```python
from build123d import *

# Parameters (mm, degrees)
F0_W          = 52
F0_H          = 1.2
F0_H_2        = 200.6
F1_DEPTH      = 50
F0_W_2        = 36.4451892475
F2_DEPTH      = 44
F0_W_3        = 531.5548107525
F3_DEPTH      = 30
F4_DEPTH      = 1.2
F5_R          = 1.2
F6_R          = 3
F7_W          = 30.6323694531
F7_H          = 5.0316524575
F8_DEPTH      = 25
F9_W          = 30.6323694531
F9_H          = 8.4860329516
F10_DEPTH     = 2
F11_T1_DEPTH  = 44.7745050768
F11_T6_DEPTH  = 22.6281685754
F11_T11_DEPTH = 22.6281685754


# Not quite as in the source:
# - a fillet or chamfer that OpenCascade refuses, or shapes differently, is made with other operations: its cross-section is extruded or revolved along the edge and cut away or added


with BuildPart() as f1:
    # F0 (on Top) → F1 (new body)
    with BuildSketch(Plane.XY):
        with Locations((-71.6174369702, 163.7731539965)):
            Rectangle(F0_W, F0_H)
        with Locations((-71.6174369702, 62.8731539965)):
            Rectangle(F0_W, F0_H_2)
        with Locations((-71.6174369702, -38.0268460035)):
            Rectangle(F0_W, F0_H)
    extrude(amount=F1_DEPTH)

    # F0 (on Top) → F2 (join)
    with BuildSketch(Plane.XY):
        with Locations((-27.3948423465, -38.0268460035)):
            Rectangle(F0_W_2, F0_H)
        with Locations((-27.3948423465, 163.7731539965)):
            Rectangle(F0_W_2, F0_H)
    extrude(amount=F2_DEPTH)

    # F0 (on Top) → F3 (join)
    with BuildSketch(Plane.XY):
        with Locations((256.6051576535, 163.7731539965)):
            Rectangle(F0_W_3, F0_H)
        with Locations((256.6051576535, -38.0268460035)):
            Rectangle(F0_W_3, F0_H)
    extrude(amount=F3_DEPTH)

    # F0 (on Top) → F4 (join)
    with BuildSketch(Plane.XY):
        with Locations((256.6051576535, 62.8731539965)):
            Rectangle(F0_W_3, F0_H_2)
        with Locations((-27.3948423465, 62.8731539965)):
            Rectangle(F0_W_2, F0_H_2)
    extrude(amount=F4_DEPTH)

    # F5
    f5_edges = [f1.edges().sort_by_distance(p)[0] for p in [
        (-71.617437, -38.626846, 50),
        (-71.617437, 164.373154, 50),
        (-97.617437, 62.873154, 50),
        (-97.617437, 62.873154, 0),
        (-45.617437, 62.873154, 50),
        (-45.617437, -38.026846, 44),
    ]]
    fillet(f5_edges, radius=F5_R)

    # F6
    f6_edges = [f1.edges().sort_by_distance(p)[0] for p in [
        (-9.172248, -38.026846, 44),
        (522.382563, -38.026846, 30),
        (522.382563, 163.773154, 30),
        (-9.172248, 163.773154, 44),
        (-9.172248, 163.773154, 30),
        (-9.172248, -38.026846, 30),
    ]]
    fillet(f6_edges, radius=F6_R)

    # F7 (on face) → F8 (cut)
    with BuildSketch(Plane.XZ.offset(-163.1731539965)):
        with Locations((11.9725436671, 3.6928627233)):
            Rectangle(F7_W, F7_H)
    extrude(amount=-F8_DEPTH, mode=Mode.SUBTRACT)

    # F9 (on face) → F10 (join)
    with BuildSketch(Plane.XZ.offset(-163.1731539965)):
        with Locations((11.9725436671, 10.4517054278)):
            Rectangle(F9_W, F9_H)
    extrude(amount=F10_DEPTH)

    # F11: fillet of radius 3 on 3 edges, made by hand

    # F11_s2 → F11_t1 (cut)
    with BuildSketch(Plane.YZ.offset(-10.4147088713)):
        with BuildLine():
            ThreePointArc((163.1731539965, 14.6947219037), (161.7236642537, 13.5983455865), (161.1731539965, 11.8662947789))
            Line((161.1731539965, 11.8662947789), (161.1731539965, 14.6947219037))
            Line((161.1731539965, 14.6947219037), (163.1731539965, 14.6947219037))
        make_face()
    extrude(amount=F11_T1_DEPTH, mode=Mode.SUBTRACT)


with BuildPart() as f11_tool4:
    # F11_s5 → F11_t6 (new body)
    with BuildSketch(Plane.XY.offset(-0.8623788598)):
        with BuildLine():
            ThreePointArc((27.2887283936, 163.1731539965), (26.1923520764, 161.7236642537), (24.4603012689, 161.1731539965))
            Line((24.4603012689, 161.1731539965), (27.2887283936, 161.1731539965))
            Line((27.2887283936, 161.1731539965), (27.2887283936, 163.1731539965))
        make_face()
    extrude(amount=F11_T6_DEPTH)

    split(bisect_by=Plane.XY.offset(1.2), keep=Keep.TOP)


with BuildPart() as f1_1:
    add(f1.part)

    # F11_t3: cut F11_tool4
    add(f11_tool4.part, mode=Mode.SUBTRACT)


with BuildPart() as f11_tool9:
    # F11_s10 → F11_t11 (new body)
    with BuildSketch(Plane.XY.offset(21.7657897155)):
        with BuildLine():
            ThreePointArc((-3.3436410595, 163.1731539965), (-2.2472647423, 161.7236642537), (-0.5152139347, 161.1731539965))
            Line((-0.5152139347, 161.1731539965), (-3.3436410595, 161.1731539965))
            Line((-3.3436410595, 161.1731539965), (-3.3436410595, 163.1731539965))
        make_face()
    extrude(amount=-F11_T11_DEPTH)

    split(bisect_by=Plane.XY.offset(1.2), keep=Keep.TOP)


with BuildPart() as f1_2:
    add(f1_1.part)

    # F11_t8: cut F11_tool9
    add(f11_tool9.part, mode=Mode.SUBTRACT)


solid = f1_2.part
```
Here's how the part is built. I have some questions about the finished solid (model axes, mm). A direction names the side the tool comes from. Give positions to 0.01 mm unless a question says otherwise; leave off trailing zeros. Write each loop counter-clockwise with the first axis right and the second up, starting at its lowest first coordinate (ties: lowest second). Pieces come first, ordered by that corner, then holes. Notation, with made-up numbers: (-18.5, -37) -> (-11.5, -37) arc R22 cw to (-11.5, -26) -> close; hole circle Ø5 at (71.25, 73). An arc over 180 degrees is marked (long way). Use one line per item in the form item = value.
1) We'd pull the mould along Y, two halves only. Please class faces 1 (the face through (522.383, 62.4, 0.4)), 2 (the face through (-45.617, 61, 25)), 3 (the face through (208, -38.627, 19)): +Y half, -Y half, draft (parallel to the pull), parting line (faces both ways), or undercut.
Verdict:
face_1 = draft
face_2 = undercut
face_3 = -Y half
2) Suppose I cut it at B-B (x = 60.5). Please give me the cut outline in (y, z).
Verdict:
outline = (-38.63, 0) -> (164.37, 0) -> (164.37, 30) -> (163.17, 30) -> (163.17, 1.2) -> (-37.43, 1.2) -> (-37.43, 30) -> (-38.63, 30) -> close
3) I'm going to push flat-ended pins straight in: pin 1 (1 mm diameter, centred on y = -38, z = 37.5, fed in from +X); pin 2 (0.6 mm diameter, centred on x = 8, y = 164, fed in from +Z); pin 3 (6 mm diameter, centred on y = 21, z = 34, fed in from +X). Where does each tip first touch, or does it pass through?
Verdict:
pin_1 = -9.17
pin_2 = 30
pin_3 = -45.62
4) If I drill on L1, parallel to Y at x = 315.5, z = 12; L2, parallel to X at y = 112, z = 34.5; L3, parallel to Z at x = 110, y = 87, over which ranges is the centre line in solid material (lowest first)? Write a range as [from, to].
Verdict:
L1 = [-38.63, -37.43], [163.17, 164.37]
L2 = [-97.62, -45.62]
L3 = [0, 1.2]
5) Suppose I cut it at A-A (y = 19.5). Please give me the cut outline in (x, z), and give its area (3 significant figures).
Verdict:
outline = (-97.62, 1.2) arc R1.2 ccw to (-96.42, 0) -> (522.38, 0) -> (522.38, 1.2) -> (-45.62, 1.2) -> (-45.62, 48.8) arc R1.2 ccw to (-46.82, 50) -> (-96.42, 50) arc R1.2 ccw to (-97.62, 48.8) -> close
area = 3,280 mm2
6) On a 3-axis mill with a long thin cutter (end or side, diameter ignored), from which of +Z, -Z, +X, -X, +Y, -Y can I reach the whole of each face in a straight line? I mean faces 4 (the face through (-72, 64, 50)), 5 (the face through (234, -37.427, 18)). Say none if no direction works.
Verdict:
face_4 = +Z, +X, -X, +Y, -Y
face_5 = +Z, +X
